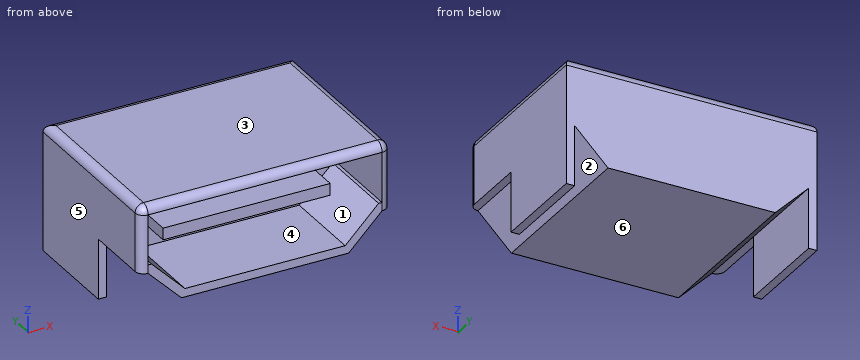
```python
from build123d import *

# Parameters (mm, degrees)
F1_DEPTH = 10.5
F3_DEPTH = 5
F4_W     = 10
F4_H     = 0.7
F5_DEPTH = 3
F6_W     = 0.5
F6_H     = 6
F7_DEPTH = 3.6
F8_R     = 0.49999


# Not quite as in the source:
# - a fillet or chamfer is up to 0.001 mm smaller than in the source, because OpenCascade refuses the exact size


with BuildPart() as f1:
    # F0 (on Front) → F1 (new body)
    with BuildSketch(Plane.XZ):
        Polygon((15, 6), (0, 6), (0, 2), (0.5, 2), (2.5, 0), (12.5, 0), (14.5, 2), (15, 2), align=None)
    extrude(amount=F1_DEPTH)

    # F2 (on face) → F3 (cut)
    with BuildSketch(Plane.XZ.offset(10.5)):
        Polygon((14.5, 5.5), (0.5, 5.5), (0.5, 2.5), (0.7071067812, 2.5), (2.7071067812, 0.5), (12.2928932188, 0.5), (14.2928932188, 2.5), (14.5, 2.5), align=None)
    extrude(amount=-F3_DEPTH, mode=Mode.SUBTRACT)

    # F4 (on face) → F5 (join)
    with BuildSketch(Plane.XZ.offset(5.5)):
        with Locations((7.5, 2.85)):
            Rectangle(F4_W, F4_H)
    extrude(amount=F5_DEPTH)

    # F6 (on face) → F7 (join)
    with BuildSketch(Plane(origin=(0, 0, 2), x_dir=(1, 0, 0), z_dir=(0, 0, -1))):
        with Locations((0.25, 3)):
            Rectangle(F6_W, F6_H)
        with Locations((14.75, 3)):
            Rectangle(F6_W, F6_H)
    extrude(amount=F7_DEPTH)

    # F8 (radius 0.5 in the source; OpenCascade refuses exactly that, so slightly less here)
    f8_edges = [f1.edges().sort_by_distance(p)[0] for p in [
        (0, -5.25, 6),
        (7.5, 0, 6),
        (15, -5.25, 6),
        (7.5, -10.5, 6),
        (0, -10.5, 4),
        (15, -10.5, 4),
    ]]
    fillet(f8_edges, radius=F8_R)


solid = f1.part
```
Part model, mm, in its own coordinate system. Face numbers are marked on the shaded views. A direction names the side the tool comes from. Round coordinates to 2 decimals unless told otherwise and drop trailing zeros. Loops run counter-clockwise (first coordinate to the right, second up) from the corner with the lowest first, then second, coordinate; pieces in that order, holes last. Notation, with made-up numbers: (-29, 41) -> (29, 41) arc R21 ccw to (29, 47) -> close; hole circle Ø6 at (16, -28). An arc over 180 degrees is marked (long way). Use a Markdown table: item, result.
1) Probe line 1 (Z direction, x = 8, y = -6); line 2 (X direction, y = -6, z = 2.75); line 3 (X direction, y = -9, z = 4.25). List the from-to ranges inside material, lowest first. Write a range as [from, to].
The answers:
| item | result |
|---|---|
| line 1 | z = [0, 0.5], [2.5, 3.2], [5.5, 6] |
| line 2 | x = [0, 0.5], [2.5, 12.5], [14.5, 15] |
| line 3 | x = [0, 0.5], [14.5, 15] |
2) Tool access for the marked faces 1, 2 and 3: list every direction of +Z, -Z, +X, -X, +Y, -Y with a clear straight run to the whole face (end or side of a thin tool).
The answers:
| item | result |
|---|---|
| face 1 | -Y |
| face 2 | -Z, +Y, -Y |
| face 3 | +Z, +X, -X, +Y, -Y |
3) Cut at A-A, the plane y = -8. List the corners of the cut face in (x, z).
The answers:
| item | result |
|---|---|
| outline | (0, 2) -> (0.5, 2) -> (2.5, 0) -> (12.5, 0) -> (14.5, 2) -> (15, 2) -> (15, 5.5) arc R0.5 ccw to (14.5, 6) -> (0.5, 6) arc R0.5 ccw to (0, 5.5) -> close; (2.5, 2.5) -> (12.5, 2.5) -> (12.5, 3.2) -> (2.5, 3.2) -> close; hole (0.5, 2.5) -> (0.71, 2.5) -> (2.71, 0.5) -> (12.29, 0.5) -> (14.29, 2.5) -> (14.5, 2.5) -> (14.5, 5.5) -> (0.5, 5.5) -> close |
4) Pull direction Z, two halves, no side cores. Call the marked faces 4, 5 and 6: pulls with the +Z half, pulls with the -Z half, needs draft (parallel to the pull), parting line crosses it, or undercut.
The answers:
| item | result |
|---|---|
| face 4 | undercut |
| face 5 | needs draft |
| face 6 | pulls with the -Z half |
5) Cut at B-B, the plane z = -0.75. List the corners of the cut face in (x, y), and give its area (3 significant figures).
The answers:
| item | result |
|---|---|
| outline | (0, -6) -> (0.5, -6) -> (0.5, 0) -> (0, 0) -> close; (14.5, -6) -> (15, -6) -> (15, 0) -> (14.5, 0) -> close |
| area | 6.00 mm2 |
6) Drop flat-ended pins along their axis: pin 1 Ø0.6 at (x, z) = (0, 0.5) entering from -Y; pin 2 Ø2.5 at (x, z) = (10, 3) entering from -Y; pin 3 Ø4 at (x, z) = (11.5, 5) entering from -Y; pin 4 Ø1.5 at (x, y) = (6.5, -7.5) entering from -Z. Give the stop position or say it passes through.
The answers:
| item | result |
|---|---|
| pin 1 | stops at y = -6 |
| pin 2 | stops at y = -8.5 |
| pin 3 | stops at y = -10.5 |
| pin 4 | stops at z = 0 |
